```python
from build123d import *

# Parameters (mm, degrees)
BOSS_EXTRUDE1_DEPTH = 2.64
SKETCH2_W           = 450.7
SKETCH2_H           = 2.2
BOSS_EXTRUDE2_DEPTH = 155.6
BOSS_EXTRUDE3_DEPTH = 105.6


with BuildPart() as part:
    # Sketch1 → Boss-Extrude1 (new body)
    with BuildSketch(Plane(origin=(0, 0, 0), x_dir=(1, 0, 0), z_dir=(0, 1, 0))):
        Polygon((-225.35, 287.45), (-225.35, -266.2), (-204.1, -266.2), (204.1, -266.2), (225.35, -266.2), (225.35, 287.45), align=None)
    extrude(amount=BOSS_EXTRUDE1_DEPTH)

    # Sketch2 → Boss-Extrude2 (add)
    with BuildSketch(Plane(origin=(0, 2.64, 0), x_dir=(1, 0, 0), z_dir=(0, 1, 0))):
        with Locations((0, -265.1)):
            Rectangle(SKETCH2_W, SKETCH2_H)
    extrude(amount=BOSS_EXTRUDE2_DEPTH)

    # Sketch3 → Boss-Extrude3 (add)
    with BuildSketch(Plane(origin=(0, 2.64, 0), x_dir=(1, 0, 0), z_dir=(0, 1, 0))):
        Polygon((1.1, -264), (1.1, 0), (202.6, 0), (202.6, 2.2), (1.1, 2.2), (1.1, 266.2), (-1.1, 266.2), (-1.1, 2.2), (-202.6, 2.2), (-202.6, 0), (-1.1, 0), (-1.1, -264), align=None)
    extrude(amount=BOSS_EXTRUDE3_DEPTH)


solid = part.part
```
Could you check a few things on this model? Use its own coordinates, in mm. A direction names the side the tool comes from. Coordinates: 2 decimals unless noted, no trailing zeros. Write each loop counter-clockwise with the first axis right and the second up, starting at its lowest first coordinate (ties: lowest second). Pieces come first, ordered by that corner, then holes. Notation, with made-up numbers: (89.5, 13.25) -> (142.5, 13.25) arc R16 ccw to (142.5, 33.25) -> close; hole circle Ø3 at (44.5, 39.5). An arc over 180 degrees is marked (long way). One line per question, with ' | ' between items. Start each with the question number.
1. If we section it at C-C (z = -193.5): Please give me the cut outline in (x, y).
2. If we section it at D-D (y = 130.5): Please give me the cut outline in (x, z).
3. If we section it at B-B (y = 34.5): Please give me the cut outline in (x, z).
4. Will these pins go through, and if not, where does the flat tip stop? P1, Ø4, axis at x = 14.5, z = 131.5, coming from the +Y side; P2, Ø1.5, axis at y = 68.5, z = -210.5, coming from the -X side; P3, Ø2.5, axis at y = 43, z = -1, coming from the +X side.
5. For faces 1 (the face through (-1.1, 55, -136)), 2 (the face through (1.1, 55, 134)), 3 (the face through (-3, 79, 264)), which set-ups out of +Z, -Z, +X, -X, +Y, -Y let a thin tool reach every point of the face, with its end or its side?
6. Please list where these lines run through material, in increasing order: line 1 along Z through (x, y) = (-33, 22.5); line 2 along Y through (x, z) = (65, 95); line 3 along Z through (x, y) = (167, 131).
7. If we section it at A-A (x = -51.5): Please give me the cut outline in (y, z), and give its area (3 significant figures).
Return value:
1) outline: (-225.35, 0) -> (225.35, 0) -> (225.35, 2.64) -> (1.1, 2.64) -> (1.1, 108.24) -> (-1.1, 108.24) -> (-1.1, 2.64) -> (-225.35, 2.64) -> close
2) outline: (-225.35, 264) -> (225.35, 264) -> (225.35, 266.2) -> (-225.35, 266.2) -> close
3) outline: (-225.35, 264) -> (-1.1, 264) -> (-1.1, 0) -> (-202.6, 0) -> (-202.6, -2.2) -> (-1.1, -2.2) -> (-1.1, -266.2) -> (1.1, -266.2) -> (1.1, -2.2) -> (202.6, -2.2) -> (202.6, 0) -> (1.1, 0) -> (1.1, 264) -> (225.35, 264) -> (225.35, 266.2) -> (-225.35, 266.2) -> close
4) P1: stops at y = 2.64 | P2: stops at x = -1.1 | P3: stops at x = 202.6
5) face 1: -Z, -X, +Y | face 2: +X, +Y | face 3: +Y
6) line 1: z = -2.2 to 0, 264 to 266.2 | line 2: y = 0 to 2.64 | line 3: z = 264 to 266.2
7) outline: (0, -287.45) -> (2.64, -287.45) -> (2.64, -2.2) -> (108.24, -2.2) -> (108.24, 0) -> (2.64, 0) -> (2.64, 264) -> (158.24, 264) -> (158.24, 266.2) -> (0, 266.2) -> close | area: 2,040 mm²
